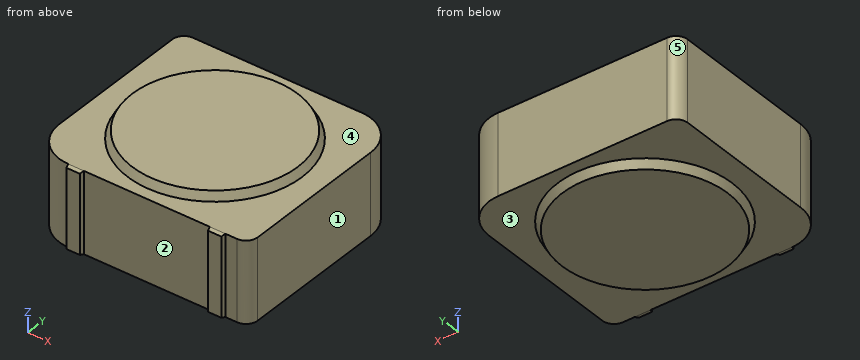
```python
from build123d import *

# Parameters (mm, degrees)
SKETCH1_W                     = 281.9
SKETCH1_H                     = 254
BOSS_EXTRUDE1_DEPTH           = 104
SKETCH3_R                     = 112
BOSS_EXTRUDE3_DEPTH           = 10
BOSS_EXTRUDE3_TAPER           = 30
SKETCH5_R                     = 112
BOSS_EXTRUDE5_DEPTH           = 10
BOSS_EXTRUDE5_TAPER           = 30
FILLET5_R                     = 50
FILLET7_R                     = 15
FILLET8_R                     = 15
FILLET9_R                     = 50
SKETCH6_W                     = 20
SKETCH6_H                     = 104
BOSS_EXTRUDE7_DEPTH           = 5
BOSS_EXTRUDE7_DRAFT           = 15
BOSS_EXTRUDE7_PROFILE_2_DEPTH = 5
BOSS_EXTRUDE7_PROFILE_2_DRAFT = 15


with BuildPart() as part:
    # Sketch1 → Boss-Extrude1 (new body)
    with BuildSketch(Plane.XY):
        with Locations((140.95, 127)):
            Rectangle(SKETCH1_W, SKETCH1_H)
    extrude(amount=BOSS_EXTRUDE1_DEPTH)

    # Sketch3 → Boss-Extrude3 (add)
    with BuildSketch(Plane.XY.offset(104)):
        with Locations((140.95, 127)):
            Circle(SKETCH3_R)
    extrude(amount=BOSS_EXTRUDE3_DEPTH, taper=BOSS_EXTRUDE3_TAPER)

    # Sketch5 → Boss-Extrude5 (add)
    with BuildSketch(Plane(origin=(0, 0, 0), x_dir=(-1, 0, 0), z_dir=(0, 0, -1))):
        with Locations((-140.95, 127)):
            Circle(SKETCH5_R)
    extrude(amount=BOSS_EXTRUDE5_DEPTH, taper=BOSS_EXTRUDE5_TAPER)

    # Fillet5
    fillet5_edges = [part.edges().sort_by_distance(p)[0] for p in [
        (281.9, 254, 52),
    ]]
    fillet(fillet5_edges, radius=FILLET5_R)

    # Fillet7
    fillet7_edges = [part.edges().sort_by_distance(p)[0] for p in [
        (0, 254, 52),
    ]]
    fillet(fillet7_edges, radius=FILLET7_R)

    # Fillet8
    fillet8_edges = [part.edges().sort_by_distance(p)[0] for p in [
        (281.9, 0, 52),
    ]]
    fillet(fillet8_edges, radius=FILLET8_R)

    # Fillet9
    fillet9_edges = [part.edges().sort_by_distance(p)[0] for p in [
        (0, 0, 52),
    ]]
    fillet(fillet9_edges, radius=FILLET9_R)


with BuildPart() as boss_extrude7_tool:
    # Sketch6 → Boss-Extrude7 (with draft: the straight prism first)
    with BuildSketch(Plane.XZ):
        with Locations((241.9, 52)):
            Rectangle(SKETCH6_W, SKETCH6_H)
    extrude(amount=BOSS_EXTRUDE7_DEPTH)
    # Boss-Extrude7: the draft: its side faces are tilted about the plane it starts from
    boss_extrude7_sides = [boss_extrude7_tool.faces().sort_by_distance(p)[0] for p in [
        (241.9, -2.5, 104),
        (231.9, -2.5, 52),
        (241.9, -2.5, 0),
        (251.9, -2.5, 52),
    ]]
    draft(boss_extrude7_sides, Plane.XZ, BOSS_EXTRUDE7_DRAFT)


with BuildPart() as part_1:
    add(part.part)

    # Boss-Extrude7: add boss_extrude7_tool
    add(boss_extrude7_tool.part)


with BuildPart() as boss_extrude7_profile_2_tool:
    # Sketch6 → Boss-Extrude7 profile 2 (with draft: the straight prism first)
    with BuildSketch(Plane.XZ):
        with Locations((60, 52)):
            Rectangle(SKETCH6_W, SKETCH6_H)
    extrude(amount=BOSS_EXTRUDE7_PROFILE_2_DEPTH)
    # Boss-Extrude7 profile 2: the draft: its side faces are tilted about the plane it starts from
    boss_extrude7_profile_2_sides = [boss_extrude7_profile_2_tool.faces().sort_by_distance(p)[0] for p in [
        (50, -2.5, 52),
        (60, -2.5, 0),
        (70, -2.5, 52),
        (60, -2.5, 104),
    ]]
    draft(boss_extrude7_profile_2_sides, Plane.XZ, BOSS_EXTRUDE7_PROFILE_2_DRAFT)


with BuildPart() as part_2:
    add(part_1.part)

    # Boss-Extrude7 profile 2: add boss_extrude7_profile_2_tool
    add(boss_extrude7_profile_2_tool.part)


solid = part_2.part
```
For this review, take the finished solid that the model builds, in its own axes (mm). Face numbers are marked on the shaded views. A direction names the side the tool comes from. Coordinates: 2 decimals unless noted, no trailing zeros. Write each loop counter-clockwise with the first axis right and the second up, starting at its lowest first coordinate (ties: lowest second). Pieces come first, ordered by that corner, then holes. Notation, with made-up numbers: (56.25, 79) - (65.25, 79) arc R36 ccw to (65.25, 113) - close; hole circle Ø8 at (0.25, -33). An arc over 180 degrees is marked (long way). Put each result on its own line as item: value.
1. Wall thickness on probe 1 along Y at (x, z) = (111.5, 38.5); probe 2 along Z at (x, y) = (92, 17); probe 3 along Y at (x, z) = (181, -1.5): over which ranges is each line inside the solid? List them lowest first.
Values found:
probe 1: 0 to 254
probe 2: 0 to 104
probe 3: 23.33 to 230.67
2. Add section A-A, the plane x = 140.95. Give the boundary of the cut face in (y, z).
Values found:
outline: (0, 0) - (15, 0) - (20.77, -10) - (233.23, -10) - (239, 0) - (254, 0) - (254, 104) - (239, 104) - (233.23, 114) - (20.77, 114) - (15, 104) - (0, 104) - close
3. Mouldability with a two-part tool opening along X and no side actions: class the marked faces 1, 2 and 3 as released by +X, released by -X, zero draft, split by the parting line, or undercut.
Values found:
face 1: released by +X
face 2: undercut
face 3: zero draft
4. Machinability: for the marked faces 4 and 5, which of the approach directions +Z, -Z, +X, -X, +Y, -Y give a long, thin tool a straight path to every point of the face, cutting with its end or side? Answer none if there is none.
Values found:
face 4: +Z
face 5: +Z, -Z, -X, +Y
5. For pin 1 (3 mm diameter, centred on y = 32.5, z = 40, fed in from -X); pin 2 (2 mm diameter, centred on y = 219.5, z = 5.5, fed in from +X); pin 3 (7.5 mm diameter, centred on x = 262.5, z = 27.5, fed in from -Y), all flat-tipped, find the tip position at first contact; note any pin that passes through.
Values found:
pin 1: x = 2.63
pin 2: x = 279.75
pin 3: y = 0
6. Add section B-B, the plane z = 9. Give the boundary of the cut face in (x, y).
Values found:
outline: (0, 50) arc R50 ccw to (50, 0) - (51.34, -5) - (68.66, -5) - (70, 0) - (231.9, 0) - (233.24, -5) - (250.56, -5) - (251.9, 0) - (266.9, 0) arc R15 ccw to (281.9, 15) - (281.9, 204) arc R50 ccw to (231.9, 254) - (15, 254) arc R15 ccw to (0, 239) - close
7. Add section C-C, the plane x = 262. Give the boundary of the cut face in (y, z), then the cut area to 3 significant figures.
Values found:
outline: (0, 0) - (243.92, 0) - (243.92, 104) - (0, 104) - close
area: 25,400 mm²
